from build123d import *

# Parameters (mm, degrees)
EXTRUDE_1_DEPTH = 4


with BuildPart() as part:
    # 草图1 → 凸台-拉伸1 (new body)
    with BuildSketch(Plane(origin=(0, 0, 0), x_dir=(1, 0, 0), z_dir=(0, 1, 0))):
        with BuildLine():
            Line((-171.971094603, -45.598997709), (-166.188191845, -6.627261728))
            Line((-166.188191845, -6.627261728), (-164.805323794, -6.627261728))
            Line((-164.805323794, -6.627261728), (-158.040783066, 38.959860567))
            Line((-158.040783066, 38.959860567), (-152.108080781, 38.959860567))
            Line((-152.108080781, 38.959860567), (-152.108080781, 37.24737007))
            Line((-152.108080781, 37.24737007), (-148.462337738, 37.24737007))
            Line((-148.462337738, 37.24737007), (-148.462337738, 32.847335362))
            Line((-148.462337738, 32.847335362), (-143.936587753, 32.847335362))
            add(Edge.make_bspline(
                [(-143.936587753, 32.847335362), (-145.689971567, 27.988679884), (-153.862596813, 33.234755139), (-154.119525219, 26.561571494)],
                knots=[0, 0, 0, 0, 1, 1, 1, 1], degree=3))
            Line((-154.119525219, 26.561571494), (-159.27385159, -6.627261728))
            Line((-159.27385159, -6.627261728), (-53.798733888, -6.627261728))
            Line((-53.798733888, -6.627261728), (-59.078775537, 26.561571494))
            add(Edge.make_bspline(
                [(-68.884567171, 32.847335362), (-67.18347063, 28.238626072), (-59.875334598, 32.556519598), (-59.078775537, 26.561571494)],
                knots=[0, 0, 0, 0, 1, 1, 1, 1], degree=3))
            Line((-68.884567171, 32.847335362), (-64.233101908, 32.847335362))
            Line((-64.233101908, 32.847335362), (-64.233101908, 37.24737007))
            Line((-64.233101908, 37.24737007), (-60.587358865, 37.24737007))
            Line((-60.587358865, 37.24737007), (-60.587358865, 38.959860567))
            Line((-60.587358865, 38.959860567), (-55.684463048, 38.959860567))
            Line((-55.684463048, 38.959860567), (-48.392976961, -6.627261728))
            Line((-48.392976961, -6.627261728), (-46.758678356, -6.627261728))
            Line((-46.758678356, -6.627261728), (-40.525298042, -45.598997709))
            add(Edge.make_bspline(
                [(-40.525298042, -45.598997709), (-37.332682932, -70.815101754), (-60.587358865, -85.098918409)],
                knots=[0, 0, 0, 1, 1, 1], degree=2))
            Line((-60.587358865, -85.098918409), (-101.024567621, -102.65158724))
            Line((-101.024567621, -102.65158724), (-101.024567621, -51.689651756))
            Line((-101.024567621, -51.689651756), (-109.024567621, -51.689651756))
            Line((-109.024567621, -51.689651756), (-109.024567621, -102.65158724))
            Line((-109.024567621, -102.65158724), (-152.108080781, -85.098918409))
            add(Edge.make_bspline(
                [(-171.971094603, -45.598997709), (-176.165938526, -72.054975501), (-152.108080781, -85.098918409)],
                knots=[0, 0, 0, 1, 1, 1], degree=2))
        make_face()
    extrude(amount=EXTRUDE_1_DEPTH)


solid = part.part
Check sheet for the modelled part. Datum: model origin and axes. Units: mm. A direction names the side the tool comes from. Round coordinates to 2 decimals unless told otherwise and drop trailing zeros. Order: outer loops, then holes, each group sorted by start corner. A loop starts at its lowest first (then second) coordinate and runs counter-clockwise, first axis right, second up. Notation, with made-up numbers: M 13,57.5 L 20,57.5 A18 ccw 20,73.5 Z; hole C 58.25,71 d11. An arc over 180 degrees is marked long. One line per item, written item: value. Start each with the question number.
1. Section check A-A on z = -15.5. Enter the section's corners in (x, y).
2. Section check D-D on z = 21. Enter the section's corners in (x, y).
3. Section check B-B on x = -92. Enter the section's corners in (y, z).
4. Access from +Z, -Z, +X, -X, +Y, -Y to the whole of each face (thin tool, end or side, straight path). Record for faces 1 (the flat face through (-150, 2, -37.247)), 2 (the flat face through (-105, 2, 51.69)), 3 (the flat face through (-156.66, 1.97, -10.2)), 4 (the flat face through (-130.26, 1.97, 94)).
5. Section check C-C on z = 90.5. Enter the section's corners in (x, y).
6. Gauge pin test, flat ends, axial feed: P1, Ø1.8, axis at x = -151, y = 1, coming from the -Z side; P2, Ø0.8, axis at x = -47.5, y = 2.5, coming from the -Z side; P3, Ø1.5, axis at y = 0.5, z = 39, coming from the -X side. Record the tip position at first contact, or that the pin passes through.
7. Release check for a two-part mould opening along Z. For faces 5 (the flat face through (-161.47, 1.97, -15.85)), 6 (the flat face through (-107, 2, 6.627)), 7 (the flat face through (-64.233, 2, -35)) record: released by +Z, released by -Z, zero draft, split by the parting line, or undercut.
8. Scan lines: line 1 along X through (y, z) = (3.5, -29); line 2 along Z through (x, y) = (-108.5, 0.2); line 3 along X through (y, z) = (1.15, 5). Record each from-to range of solid material in increasing order.
Results found:
1. outline: M -161.52,0 L -155.84,0 L -155.84,4 L -161.52,4 Z; M -57.32,0 L -51.93,0 L -51.93,4 L -57.32,4 Z
2. outline: M -168.32,0 L -44.46,0 L -44.46,4 L -168.32,4 Z
3. outline: M 0,6.63 L 4,6.63 L 4,98.73 L 0,98.73 Z
4. face 1: -Z, +Y, -Y
4. face 2: +Z, +Y, -Y
4. face 3: +Y, -Y
4. face 4: +Z, -X, +Y, -Y
5. outline: M -138.85,0 L -109.02,0 L -109.02,4 L -138.85,4 Z; M -101.02,0 L -73.03,0 L -73.03,4 L -101.02,4 Z
6. P1: z = -37.25
6. P2: z = 6.63
6. P3: x = -171.1
7. face 5: released by -Z
7. face 6: undercut
7. face 7: zero draft
8. line 1: -159.52 to -153.4, -60.16 to -54.09
8. line 2: 6.63 to 51.69
8. line 3: -164.56 to -159.02, -54.06 to -48.65
